Source: CAD feature listing. Evaluate the final solid. Frame: model axes, mm. A direction names the side the tool comes from. Round coordinates to 2 decimals unless told otherwise and drop trailing zeros. Loops run counter-clockwise (first coordinate to the right, second up) from the corner with the lowest first, then second, coordinate; pieces in that order, holes last. Notation, with made-up numbers: M 69,-5 L 89,-5 A13 cw 89,19 Z; hole C -32,-34.75 d1. An arc over 180 degrees is marked long. Answer as CSV lines item,"result". Start each with the question number.
```python
from build123d import *

# Parameters (mm, degrees)
SKETCH1_W           = 50.8
SKETCH1_H           = 25.4
SKETCH1_W_2         = 45.72
SKETCH1_H_2         = 20.32
EXTRUDE_THIN1_DEPTH = 398.78
SKETCH2_R           = 1.3462
CUT_EXTRUDE1_DEPTH  = 51.8
LPATTERN1_COUNT     = 19
LPATTERN1_PITCH     = 25.4
CUT_EXTRUDE2_DEPTH  = 26.4
SKETCH4_R           = 19.05
CUT_EXTRUDE3_DEPTH  = 26.4000001


with BuildPart() as part:
    # Sketch1 → Extrude-Thin1 (new body)
    with BuildSketch(Plane.XY):
        Rectangle(SKETCH1_W, SKETCH1_H)
        Rectangle(SKETCH1_W_2, SKETCH1_H_2, mode=Mode.SUBTRACT)
    extrude(amount=EXTRUDE_THIN1_DEPTH)

    # Sketch2 → Cut-Extrude1 (cut, through all)
    with BuildSketch(Plane(origin=(25.4, 0, 0), x_dir=(0, 0, -1), z_dir=(1, 0, 0))):
        with Locations((-392.43, 0)):
            Circle(SKETCH2_R)
    cut_extrude1 = extrude(amount=-CUT_EXTRUDE1_DEPTH, mode=Mode.SUBTRACT)

    # LPattern1: Cut-Extrude1 ×19
    with Locations(*[(0, 0, -i * LPATTERN1_PITCH) for i in range(1, LPATTERN1_COUNT)]):
        add(cut_extrude1, mode=Mode.SUBTRACT)

    # Sketch3 → Cut-Extrude2 (cut, through all)
    with BuildSketch(Plane(origin=(0, 12.7, 0), x_dir=(1, 0, 0), z_dir=(0, 1, 0))):
        with BuildLine():
            ThreePointArc((23.8125, -398.78), (23.595945628, -395.57586109), (22.950221268, -392.43))
            ThreePointArc((22.950221268, -392.43), (0, -374.9675), (-22.950221268, -392.43))
            ThreePointArc((-22.950221268, -392.43), (-23.595945628, -395.57586109), (-23.8125, -398.78))
            Line((-23.8125, -398.78), (23.8125, -398.78))
        make_face()
        with BuildLine():
            ThreePointArc((-23.8125, -398.78), (0, -422.5925), (23.8125, -398.78))
            Line((23.8125, -398.78), (-23.8125, -398.78))
        make_face()
        with BuildLine():
            Line((25.4, -398.78), (25.4, -392.43))
            Line((25.4, -392.43), (22.950221268, -392.43))
            ThreePointArc((22.950221268, -392.43), (23.595945628, -395.57586109), (23.8125, -398.78))
            Line((23.8125, -398.78), (25.4, -398.78))
        make_face()
        with BuildLine():
            ThreePointArc((-23.8125, -398.78), (-23.595945628, -395.57586109), (-22.950221268, -392.43))
            Line((-22.950221268, -392.43), (-25.4, -392.43))
            Line((-25.4, -392.43), (-25.4, -398.78))
            Line((-25.4, -398.78), (-23.8125, -398.78))
        make_face()
        with BuildLine():
            ThreePointArc((-20.88995587, -11.43), (0, -23.8125), (20.88995587, -11.43))
            ThreePointArc((20.88995587, -11.43), (23.07029725, -5.898859301), (23.8125, 0))
            Line((23.8125, 0), (-23.8125, 0))
            ThreePointArc((-23.8125, 0), (-23.07029725, -5.898859301), (-20.88995587, -11.43))
        make_face()
        with BuildLine():
            Line((-23.8125, 0), (23.8125, 0))
            ThreePointArc((23.8125, 0), (0, 23.8125), (-23.8125, 0))
        make_face()
        with BuildLine():
            Line((-25.4, -11.43), (-20.88995587, -11.43))
            ThreePointArc((-20.88995587, -11.43), (-23.07029725, -5.898859301), (-23.8125, 0))
            Line((-23.8125, 0), (-25.4, 0))
            Line((-25.4, 0), (-25.4, -11.43))
        make_face()
        with BuildLine():
            Line((20.88995587, -11.43), (25.4, -11.43))
            Line((25.4, -11.43), (25.4, 0))
            Line((25.4, 0), (23.8125, 0))
            ThreePointArc((23.8125, 0), (23.07029725, -5.898859301), (20.88995587, -11.43))
        make_face()
    extrude(amount=-CUT_EXTRUDE2_DEPTH, mode=Mode.SUBTRACT)

    # Sketch4 → Cut-Extrude3 (cut, through all)
    with BuildSketch(Plane(origin=(0, 12.7, 0), x_dir=(1, 0, 0), z_dir=(0, 1, 0))):
        with Locations((0, -328.93)):
            Circle(SKETCH4_R)
        with Locations((0, -74.93)):
            Circle(SKETCH4_R)
    extrude(amount=-CUT_EXTRUDE3_DEPTH, mode=Mode.SUBTRACT)


solid = part.part
```
1) Mould query, pull axis X, two halves, no side actions, for faces 3 (the flat face through (-25.4, 0, 199)), 4 (the cylindrical face through (-0.36, -11.41, 23.81)), 5 (the flat face through (0, 12.7, 199)). Classes: pulls with the +X half, pulls with the -X half, needs draft (parallel to the pull), parting line crosses it, or undercut.
2) Contact query for flat-ended pins moving along their axis: pin 1 Ø23 at (x, z) = (0, 328.93) entering from +Y; pin 2 Ø4.5 at (y, z) = (0, 62.23) entering from -X; pin 3 Ø10 at (x, y) = (-0.5, 9.5) entering from +Z. Output: stop coordinate, or through.
3) Section C-C, the plane x = 15. Return loops of the section in (y, z).
4) Section A-A, the plane z = 158. Return loops of the section in (x, y), and give its area (3 significant figures).
5) Section B-B, the plane x = 0. Return loops of the section in (y, z), and give its area (3 significant figures).
6) Ray query, line 1 along Z through (x, y) = (1, 11.75); line 2 along Y through (x, z) = (20, 290); line 3 along X through (y, z) = (1.5, 138.5). Return the intervals inside material, ascending.
7) Access query for faces 1 (the flat face through (25.4, 0, 199)), 2 (the flat face through (0, -10.16, 199)). Directions: +Z, -Z, +X, -X, +Y, -Y. A direction counts if a zero-diameter tool reaches every point of the face in a straight line with its end or side. Return the directions, or none.
Findings below:
1,face 3,"pulls with the -X half"
1,face 4,"undercut"
1,face 5,"needs draft"
2,pin 1,"through"
2,pin 2,"x = -25.4"
2,pin 3,"z = 375.6"
3,outline,"M -12.7,18.49 L -10.16,18.49 L -10.16,63.19 L -12.7,63.19 Z; M -12.7,86.67 L -10.16,86.67 L -10.16,317.19 L -12.7,317.19 Z; M -12.7,340.67 L -10.16,340.67 L -10.16,380.29 L -12.7,380.29 Z; M 10.16,18.49 L 12.7,18.49 L 12.7,63.19 L 10.16,63.19 Z; M 10.16,86.67 L 12.7,86.67 L 12.7,317.19 L 10.16,317.19 Z; M 10.16,340.67 L 12.7,340.67 L 12.7,380.29 L 10.16,380.29 Z"
4,outline,"M -25.4,-12.7 L 25.4,-12.7 L 25.4,12.7 L -25.4,12.7 Z; hole M -22.86,-10.16 L 22.86,-10.16 L 22.86,10.16 L -22.86,10.16 Z"
4,area,"361 mm²"
5,outline,"M -12.7,23.81 L -10.16,23.81 L -10.16,55.88 L -12.7,55.88 Z; M -12.7,93.98 L -10.16,93.98 L -10.16,309.88 L -12.7,309.88 Z; M -12.7,347.98 L -10.16,347.98 L -10.16,374.97 L -12.7,374.97 Z; M 10.16,23.81 L 12.7,23.81 L 12.7,55.88 L 10.16,55.88 Z; M 10.16,93.98 L 12.7,93.98 L 12.7,309.88 L 10.16,309.88 Z; M 10.16,347.98 L 12.7,347.98 L 12.7,374.97 L 10.16,374.97 Z"
5,area,"1,400 mm²"
6,line 1,"23.79 to 55.91, 93.95 to 309.91, 347.95 to 374.99"
6,line 2,"-12.7 to -10.16, 10.16 to 12.7"
6,line 3,"-25.4 to -22.86, 22.86 to 25.4"
7,face 1,"+Z, -Z, +X, +Y, -Y"
7,face 2,"+Z, -Z"
